from build123d import *

# Parameters (mm, degrees)
F0_R     = 2.75
F0_R_2   = 2
F1_DEPTH = 3
F2_DEPTH = 1.5
F4_DEPTH = 7
F6_DEPTH = 9
F7_SIZE  = 0.2


# Not quite as in the source:
# - after a boolean that leaves OpenCascade's solid faulty, fix() repairs it


with BuildPart() as f1:
    # F0 (on Top) → F1 (new body)
    with BuildSketch(Plane.XY):
        Circle(F0_R)
        Circle(F0_R_2, mode=Mode.SUBTRACT)
        Circle(F0_R_2)
    extrude(amount=-F1_DEPTH)

    # F0 (on Top) → F2 (join)
    with BuildSketch(Plane.XY):
        Circle(F0_R_2)
    extrude(amount=F2_DEPTH)

    # F3 (on face) → F4 (join)
    with BuildSketch(Plane.XY.offset(1.5)):
        with BuildLine():
            ThreePointArc((1.5, 1.3228756555), (0, 2), (-1.5, 1.3228756555))
            Line((-1.5, 1.3228756555), (-1.5, -1.3228756555))
            ThreePointArc((-1.5, -1.3228756555), (0, -2), (1.5, -1.3228756555))
            Line((1.5, -1.3228756555), (1.5, 1.3228756555))
        make_face()
    extrude(amount=F4_DEPTH)

    # F5 (on face) → F6 (join)
    with BuildSketch(Plane(origin=(0, 0, -3), x_dir=(1, 0, 0), z_dir=(0, 0, -1))):
        with BuildLine():
            ThreePointArc((0.25, -2.7386127875), (0.63122595, -2.676575013), (1, -2.5617376915))
            Line((1, -2.5617376915), (1, -1))
            Line((1, -1), (2.5617376915, -1))
            ThreePointArc((2.5617376915, -1), (2.676575013, -0.63122595), (2.7386127875, -0.25))
            ThreePointArc((2.7386127875, -0.25), (2.7471517218, -0.1251296014), (2.75, 0))
            ThreePointArc((2.75, 0), (2.7471517218, 0.1251296014), (2.7386127875, 0.25))
            ThreePointArc((2.7386127875, 0.25), (2.676575013, 0.63122595), (2.5617376915, 1))
            Line((2.5617376915, 1), (1, 1))
            Line((1, 1), (1, 2.5617376915))
            ThreePointArc((1, 2.5617376915), (0.63122595, 2.676575013), (0.25, 2.7386127875))
            ThreePointArc((0.25, 2.7386127875), (0, 2.75), (-0.25, 2.7386127875))
            ThreePointArc((-0.25, 2.7386127875), (-0.63122595, 2.676575013), (-1, 2.5617376915))
            Line((-1, 2.5617376915), (-1, 1))
            Line((-1, 1), (-2.5617376915, 1))
            ThreePointArc((-2.5617376915, 1), (-2.676575013, 0.63122595), (-2.7386127875, 0.25))
            ThreePointArc((-2.7386127875, 0.25), (-2.75, 0), (-2.7386127875, -0.25))
            ThreePointArc((-2.7386127875, -0.25), (-2.676575013, -0.63122595), (-2.5617376915, -1))
            Line((-2.5617376915, -1), (-1, -1))
            Line((-1, -1), (-1, -2.5617376915))
            ThreePointArc((-1, -2.5617376915), (-0.63122595, -2.676575013), (-0.25, -2.7386127875))
            ThreePointArc((-0.25, -2.7386127875), (0, -2.75), (0.25, -2.7386127875))
        make_face()
        with BuildLine():
            ThreePointArc((2.75, 0), (2.7471517218, -0.1251296014), (2.7386127875, -0.25))
            Line((2.7386127875, -0.25), (3.2, 0))
            Line((3.2, 0), (2.7386127875, 0.25))
            ThreePointArc((2.7386127875, 0.25), (2.7471517218, 0.1251296014), (2.75, 0))
        make_face()
        with BuildLine():
            Line((0, -3.2), (0.25, -2.7386127875))
            ThreePointArc((0.25, -2.7386127875), (0, -2.75), (-0.25, -2.7386127875))
            Line((-0.25, -2.7386127875), (0, -3.2))
        make_face()
        with BuildLine():
            Line((-3.2, 0), (-2.7386127875, -0.25))
            ThreePointArc((-2.7386127875, -0.25), (-2.75, 0), (-2.7386127875, 0.25))
            Line((-2.7386127875, 0.25), (-3.2, 0))
        make_face()
        with BuildLine():
            ThreePointArc((-0.25, 2.7386127875), (0, 2.75), (0.25, 2.7386127875))
            Line((0.25, 2.7386127875), (0, 3.2))
            Line((0, 3.2), (-0.25, 2.7386127875))
        make_face()
    extrude(amount=F6_DEPTH)

    add(f1.part.fix(), mode=Mode.REPLACE)

    # F7
    f7_edges = [f1.edges().sort_by_distance(p)[0] for p in [
        (-0.125, 2.969306, -12),
        (0.125, 2.969306, -12),
        (-2.969306, 0.125, -12),
        (-2.969306, -0.125, -12),
        (0.125, -2.969306, -12),
        (-0.125, -2.969306, -12),
        (2.969306, -0.125, -12),
        (2.969306, 0.125, -12),
    ]]
    chamfer(f7_edges, length=F7_SIZE)


solid = f1.part
Model file for the job. Use its own axes, mm. A direction names the side the tool comes from. Give positions to 0.01 mm unless a question says otherwise; leave off trailing zeros. Order: outer loops, then holes, each group sorted by start corner. A loop starts at its lowest first (then second) coordinate and runs counter-clockwise, first axis right, second up. Notation, with made-up numbers: (-9.75, 31) - (9.25, 31) arc R4 ccw to (9.25, 36) - close; hole circle Ø2 at (-31.5, 62). An arc over 180 degrees is marked (long way). Return JSON: item names as keys, results as strings.
1) 3-axis set-ups, long thin cutter, end or side, ignore diameter. For faces 1 (the flat face through (-2, 1, -7)), 2 (the flat face through (1.5, 0, 5)), 3 (the flat face through (-1.6, -1.6, -3)): which of +Z, -Z, +X, -X, +Y, -Y reach the whole face in a straight line?
Geometry says:
{"face 1": "-Z, -X, +Y", "face 2": "+Z, +X, +Y, -Y", "face 3": "-Z, -X, -Y"}
2) Flat gauge pins, fed straight in: P1, Ø1, axis at y = -0.5, z = 1.5, coming from the +X side; P2, Ø0.8, axis at x = -2, y = -2, coming from the -Z side; P3, Ø0.5, axis at x = 2, z = -9.5, coming from the -Y side; P4, Ø1.7, axis at x = -1.5, y = 1.5, coming from the -Z side. Where does each tip first touch, or does it go through?
Geometry says:
{"P1": "x = 2", "P2": "z = -3", "P3": "y = -1", "P4": "z = -12"}
3) Probe line 1 (Z direction, x = 1.75, y = 0.25); line 2 (Z direction, x = -2.25, y = -1.5); line 3 (Y direction, x = 1, z = -1). List the from-to ranges inside material, lowest first. Write a range as from..to.
Geometry says:
{"line 1": "-12..1.5", "line 2": "-3..0", "line 3": "-2.56..2.56"}
4) Cut at C-C, the plane y = -0.75. Give the cut face in (x, z), plus the area to 3 significant figures.
Geometry says:
{"outline": "(-2.65, -12) - (2.65, -12) - (2.65, 0) - (1.85, 0) - (1.85, 1.5) - (1.5, 1.5) - (1.5, 8.5) - (-1.5, 8.5) - (-1.5, 1.5) - (-1.85, 1.5) - (-1.85, 0) - (-2.65, 0) - close", "area": "90.1 mm²"}
5) Cut at B-B, the plane x = -1.25. Give the cut face in (y, z), plus the area to 3 significant figures.
Geometry says:
{"outline": "(-2.45, -3) - (-1, -3) - (-1, -12) - (1, -12) - (1, -3) - (2.45, -3) - (2.45, 0) - (1.56, 0) - (1.56, 8.5) - (-1.56, 8.5) - (-1.56, 0) - (-2.45, 0) - close", "area": "59.2 mm²"}
6) Cut at A-A, the plane z = -4. Give the cut face in (x, y).
Geometry says:
{"outline": "(-3.2, 0) - (-2.74, -0.25) arc R2.75 ccw to (-2.56, -1) - (-1, -1) - (-1, -2.56) arc R2.75 ccw to (-0.25, -2.74) - (0, -3.2) - (0.25, -2.74) arc R2.75 ccw to (1, -2.56) - (1, -1) - (2.56, -1) arc R2.75 ccw to (2.74, -0.25) - (3.2, 0) - (2.74, 0.25) arc R2.75 ccw to (2.56, 1) - (1, 1) - (1, 2.56) arc R2.75 ccw to (0.25, 2.74) - (0, 3.2) - (-0.25, 2.74) arc R2.75 ccw to (-1, 2.56) - (-1, 1) - (-2.56, 1) arc R2.75 ccw to (-2.74, 0.25) - close"}
7) Cut at D-D, the plane z = 0.75. Give the cut face in (x, y).
Geometry says:
{"outline": "circle Ø4 at (0, 0)"}
